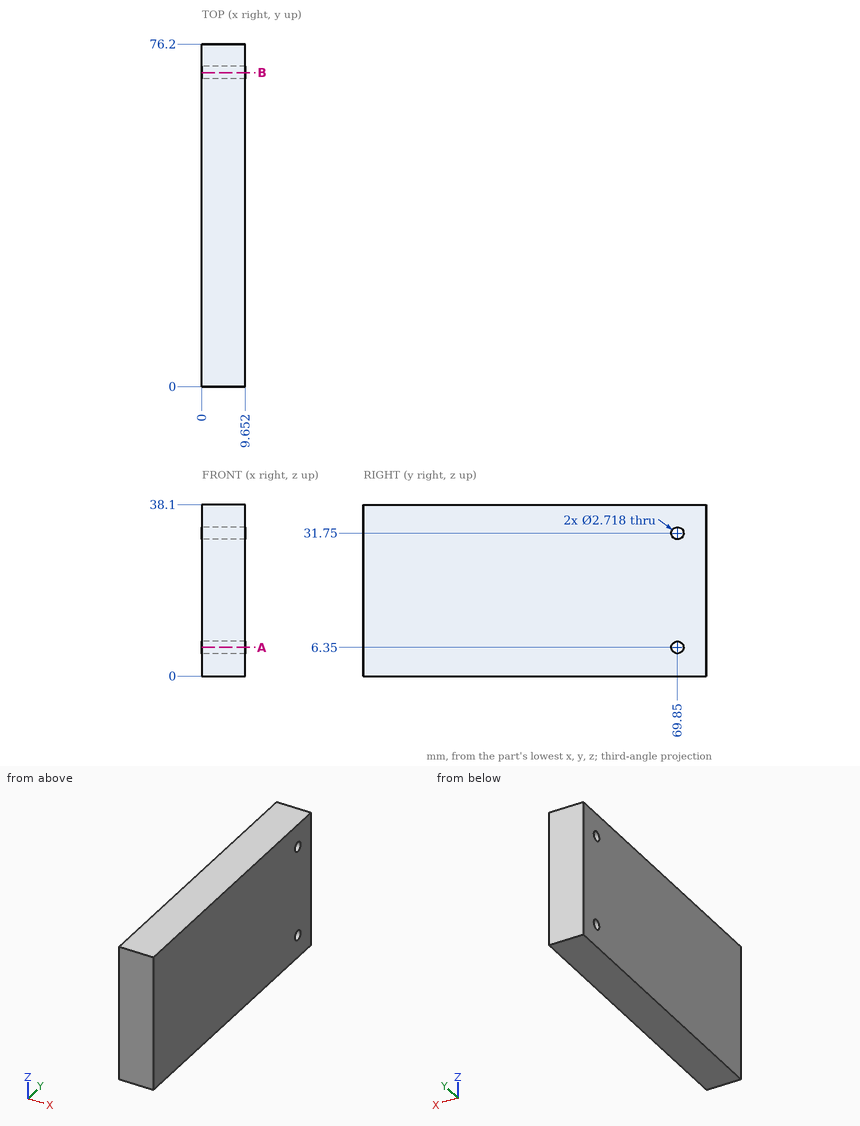
Source: three-view drawing plus pictorial views. Frame: mm from the lowest corner of the part. Round coordinates to 2 decimals unless told otherwise and drop trailing zeros. Loops run counter-clockwise (first coordinate to the right, second up) from the corner with the lowest first, then second, coordinate; pieces in that order, holes last. Notation, with made-up numbers: M 48,1 L 71,1 A28 cw 71,26 Z; hole C 65,47 d11. An arc over 180 degrees is marked long. Answer as CSV lines item,"result". Start each with the question number.
(1) First-contact query: pin 1 (1.5 mm diameter, centred on x = 6, y = 61, fed in from -Z). Flat tip, straight axial feed; report the tip coordinate or a pass-through.
(2) Section A-A, the plane z = 6.35. Output: boundary loops of the cut face in (x, y), plus the area to 3 significant figures.
(3) Section B-B, the plane y = 69.85. Output: boundary loops of the cut face in (x, z).
(4) Line query: line 1 (Z direction, x = 7, y = 69.85); line 2 (Y direction, x = 6.75, z = 31.75). Output: solid intervals per line, ascending. Write a range as [from, to].
Values found:
1,pin 1,"stops at z = 0"
2,outline,"M 0,0 L 9.65,0 L 9.65,68.49 L 0,68.49 Z; M 0,71.21 L 9.65,71.21 L 9.65,76.2 L 0,76.2 Z"
2,area,"709 mm²"
3,outline,"M 0,0 L 9.65,0 L 9.65,4.99 L 0,4.99 Z; M 0,7.71 L 9.65,7.71 L 9.65,30.39 L 0,30.39 Z; M 0,33.11 L 9.65,33.11 L 9.65,38.1 L 0,38.1 Z"
4,line 1,"z = [0, 4.99], [7.71, 30.39], [33.11, 38.1]"
4,line 2,"y = [0, 68.49], [71.21, 76.2]"
